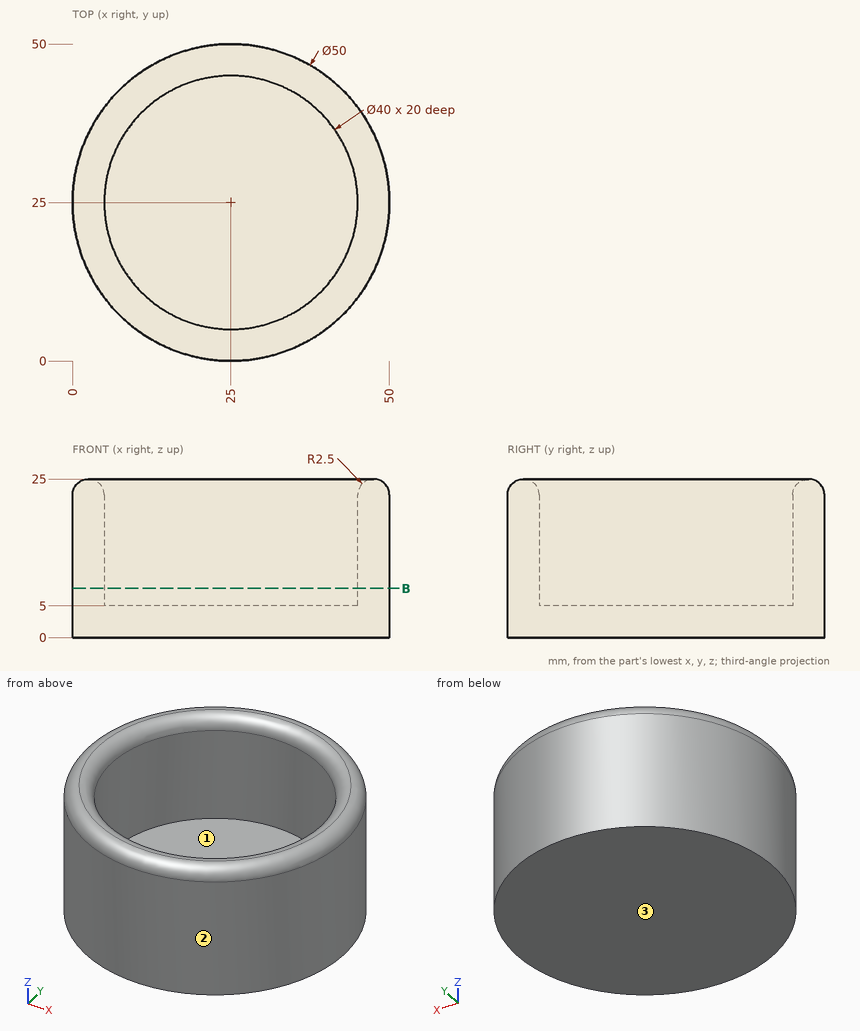
The figure shows three views and two pictorial views of one solid part (mm, origin at its lowest corner). Answer the questions. Give positions to 0.01 mm unless a question says otherwise; leave off trailing zeros. Write each loop counter-clockwise with the first axis right and the second up, starting at its lowest first coordinate (ties: lowest second). Pieces come first, ordered by that corner, then holes. Notation, with made-up numbers: (-36, 21) - (1, 21) arc R8 cw to (1, 31) - close; hole circle Ø4 at (36, 89.5). An arc over 180 degrees is marked (long way). Return JSON: item names as keys, results as strings.
Q1. Given P1, Ø1, axis at x = 40, z = 19.5, coming from the +Y side; P2, Ø6, axis at y = 18, z = 20, coming from the +X side; P3, Ø12, axis at x = 28.5, z = 10.5, coming from the +Y side, each flat-ended and moving along its own axis, determine where each tip first touches the part or whether it passes through.
Reply:
{"P1": "y = 45.37", "P2": "x = 49.68", "P3": "y = 50"}
Q2. A cutting plane is placed at B-B, the plane z = 7.75. Determine the outline of the cut face in (x, y), and give its area (3 significant figures).
Reply:
{"outline": "circle Ø50 at (25, 25); hole circle Ø40 at (25, 25)", "area": "707 mm²"}
Q3. For a pull along Y with two mould halves and no side action, classify the marked faces 1, 2 and 3 as released by +Y, released by -Y, zero draft, split by the parting line, or undercut.
Reply:
{"face 1": "undercut", "face 2": "split by the parting line", "face 3": "zero draft"}
Q4. Consider line 1 along Y through (x, z) = (25, 13.75); line 2 along Z through (x, y) = (22, 26.5); line 3 along X through (y, z) = (16, 18). Determine where each line is inside the solid, lowest interval first. Write a range as [from, to].
Reply:
{"line 1": "[0, 5], [45, 50]", "line 2": "[0, 5]", "line 3": "[1.68, 7.14], [42.86, 48.32]"}
